Verification items for the finished model (mm, model axes). Face numbers are marked on the shaded views. A direction names the side the tool comes from. Round coordinates to 2 decimals unless told otherwise and drop trailing zeros. Order: outer loops, then holes, each group sorted by start corner. A loop starts at its lowest first (then second) coordinate and runs counter-clockwise, first axis right, second up. Notation, with made-up numbers: M 63,63 L 110,63 A6 ccw 110,73 Z; hole C 59.5,-18 d7. An arc over 180 degrees is marked long. Use CSV: the item, a comma, the result in double quotes. Start each with the question number.
Q1. Scan lines: line 1 (Z direction, x = 1.75, y = 3.75); line 2 (Z direction, x = 2, y = 9); line 3 (Z direction, x = 2.5, y = 9). Record each from-to range of solid material in increasing order.
Q2. Mould release check, pull along Z, two halves, no side actions. Record for the marked faces 4, 5 and 6: +Z half, -Z half, draft (parallel to the pull), parting line (faces both ways), or undercut.
Q3. Set-up check for the marked faces 1, 2 and 3: record each of +Z, -Z, +X, -X, +Y, -Y from which the full face is reachable in a straight line by a thin tool's end or side.
Q4. Sectioned sample at B-B (x = 0.5). Enter the section's corners in (y, z).
Q5. Sectioned sample at A-A (y = 5). Enter the section's corners in (x, z).
Q6. Sectioned sample at D-D (z = 0). Enter the section's corners in (x, y), and give its area (3 significant figures).
Q7. Gauge pin test, flat ends, axial feed: pin 1 Ø3 at (y, z) = (5, -8.89) entering from +X; pin 2 Ø4.5 at (y, z) = (5, 9) entering from +X; pin 3 Ø6 at (y, z) = (3.5, -6) entering from +X. Record the tip position at first contact, or that the pin passes through.
Q8. Sectioned sample at C-C (y = 1.5). Enter the section's corners in (x, z), and give its area (3 significant figures).
```python
from build123d import *

# Parameters (mm, degrees)
EXTRUDE_1_DEPTH     = 10
SKETCH_2_R          = 1.75
CUT_EXTRUDE_1_DEPTH = 27.305892876


with BuildPart() as part:
    # 草图1 → 凸台-拉伸1 (new body)
    with BuildSketch(Plane(origin=(0, 0, 0), x_dir=(1, 0, 0), z_dir=(0, 1, 0))):
        with BuildLine():
            Line((0, 24), (0, 4))
            ThreePointArc((0, 4), (4, 0), (0, -4))
            Line((0, -4), (0, -12))
            Line((0, -12), (3, -12))
            Line((3, -12), (3, -6.32455532))
            ThreePointArc((3, -6.32455532), (7, 0), (3, 6.32455532))
            Line((3, 6.32455532), (3, 24))
            Line((3, 24), (0, 24))
        make_face()
    extrude(amount=EXTRUDE_1_DEPTH)

    # 草图2 → 切除-拉伸1 (cut, through all)
    with BuildSketch(Plane(origin=(3, 0, 0), x_dir=(0, 0, -1), z_dir=(1, 0, 0))):
        with Locations((-9.16227766, 5)):
            Circle(SKETCH_2_R)
        with Locations((8.888984546, 5)):
            Circle(SKETCH_2_R)
    extrude(amount=-CUT_EXTRUDE_1_DEPTH, mode=Mode.SUBTRACT)


solid = part.part
```
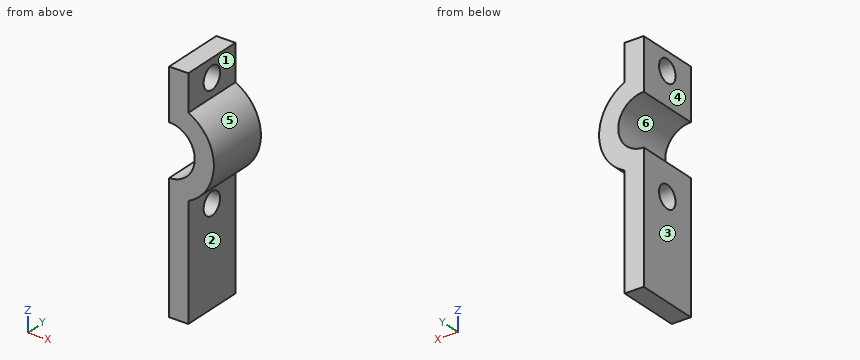
Verdict:
1,line 1,"z = -24 to -10.11, -7.66 to -3.6, 3.6 to 7.94, 10.39 to 12"
1,line 2,"z = -24 to -3.46, 3.46 to 12"
1,line 3,"z = -24 to -3.12, 3.12 to 12"
2,face 4,"draft"
2,face 5,"parting line"
2,face 6,"undercut"
3,face 1,"+Z, +X, +Y, -Y"
3,face 2,"-Z, +X, +Y, -Y"
3,face 3,"+Z, -Z, -X, +Y, -Y"
4,outline,"M 0,-24 L 10,-24 L 10,-3.97 L 0,-3.97 Z; M 0,3.97 L 10,3.97 L 10,12 L 0,12 Z; hole C 5,-8.89 d3.5; hole C 5,9.16 d3.5"
5,outline,"M 0,-24 L 3,-24 L 3,-10.64 L 0,-10.64 Z; M 0,-7.14 L 3,-7.14 L 3,-6.32 A7 ccw 3,6.32 L 3,7.41 L 0,7.41 L 0,4 A4 cw 0,-4 Z; M 0,10.91 L 3,10.91 L 3,12 L 0,12 Z"
6,outline,"M 4,0 L 7,0 L 7,10 L 4,10 Z"
6,area,"30.0 mm²"
7,pin 1,"passes through"
7,pin 2,"stops at x = 3"
7,pin 3,"stops at x = 6.32"
8,outline,"M 0,-24 L 3,-24 L 3,-6.32 A7 ccw 3,6.32 L 3,12 L 0,12 L 0,4 A4 cw 0,-4 Z"
8,area,"119 mm²"
